from build123d import *

# Parameters (mm, degrees)
SKETCH1_R           = 65
SKETCH1_R_2         = 3.75
SKETCH1_R_3         = 2.25
BOSS_EXTRUDE1_DEPTH = 2.3749


with BuildPart() as part:
    # Sketch1 → Boss-Extrude1 (new, symmetric)
    with BuildSketch(Plane.XY):
        with BuildLine():
            Line((-45.414170693, 71.792048343), (-34.829629131, 111.294095226))
            ThreePointArc((-34.829629131, 111.294095226), (-33.043807145, 113.966766701), (-30, 115))
            Line((-30, 115), (30, 115))
            ThreePointArc((30, 115), (33.043807145, 113.966766701), (34.829629131, 111.294095226))
            Line((34.829629131, 111.294095226), (45.414170693, 71.792048343))
            ThreePointArc((45.414170693, 71.792048343), (46.806677386, 68.753444104), (49.122761322, 66.343476093))
            ThreePointArc((49.122761322, 66.343476093), (82.55, 0), (49.122761322, -66.343476093))
            ThreePointArc((49.122761322, -66.343476093), (46.806677386, -68.753444104), (45.414170693, -71.792048343))
            Line((45.414170693, -71.792048343), (34.829629131, -111.294095226))
            ThreePointArc((34.829629131, -111.294095226), (33.043807145, -113.966766701), (30, -115))
            Line((30, -115), (-30, -115))
            ThreePointArc((-30, -115), (-33.043807145, -113.966766701), (-34.829629131, -111.294095226))
            Line((-34.829629131, -111.294095226), (-45.414170693, -71.792048343))
            ThreePointArc((-45.414170693, -71.792048343), (-46.806677386, -68.753444104), (-49.122761322, -66.343476093))
            ThreePointArc((-49.122761322, -66.343476093), (-82.55, 0), (-49.122761322, 66.343476093))
            ThreePointArc((-49.122761322, 66.343476093), (-46.806677386, 68.753444104), (-45.414170693, 71.792048343))
        make_face()
        Circle(SKETCH1_R, mode=Mode.SUBTRACT)
        with Locations((-20, 100)):
            Circle(SKETCH1_R_2, mode=Mode.SUBTRACT)
        with Locations((20, 100)):
            Circle(SKETCH1_R_2, mode=Mode.SUBTRACT)
        with Locations(Location((20, -100, 0), (0, 0, 180))):
            Circle(SKETCH1_R_2, mode=Mode.SUBTRACT)
        with Locations(Location((-20, -100, 0), (0, 0, 180))):
            Circle(SKETCH1_R_2, mode=Mode.SUBTRACT)
        with Locations((0, 78.74)):
            Circle(SKETCH1_R_3, mode=Mode.SUBTRACT)
        with Locations((46.282210766, 63.701998137)):
            Circle(SKETCH1_R_3, mode=Mode.SUBTRACT)
        with Locations((74.886190093, 24.331998137)):
            Circle(SKETCH1_R_3, mode=Mode.SUBTRACT)
        with Locations((74.886190093, -24.331998137)):
            Circle(SKETCH1_R_3, mode=Mode.SUBTRACT)
        with Locations((46.282210766, -63.701998137)):
            Circle(SKETCH1_R_3, mode=Mode.SUBTRACT)
        with Locations((0, -78.74)):
            Circle(SKETCH1_R_3, mode=Mode.SUBTRACT)
        with Locations((-46.282210766, -63.701998137)):
            Circle(SKETCH1_R_3, mode=Mode.SUBTRACT)
        with Locations((-74.886190093, -24.331998137)):
            Circle(SKETCH1_R_3, mode=Mode.SUBTRACT)
        with Locations((-74.886190093, 24.331998137)):
            Circle(SKETCH1_R_3, mode=Mode.SUBTRACT)
        with Locations((-46.282210766, 63.701998137)):
            Circle(SKETCH1_R_3, mode=Mode.SUBTRACT)
    extrude(amount=BOSS_EXTRUDE1_DEPTH, both=True)


solid = part.part
Read the model definition and answer for the solid it produces. Units are mm, in the model's axes. Coordinates: 2 decimals unless noted, no trailing zeros. Loops run counter-clockwise (first coordinate to the right, second up) from the corner with the lowest first, then second, coordinate; pieces in that order, holes last. Notation, with made-up numbers: (11.5, -28) - (58.5, -28) arc R29 ccw to (58.5, -3) - close; hole circle Ø3 at (16.5, 34). An arc over 180 degrees is marked (long way). Answer in a Markdown table with one row per item.
Q1. Find section B-B on x = 20. Write down the section's boundary in (y, z), plus the area to 3 significant figures.
Here are the results:
| item | result |
|---|---|
| outline | (-115, -2.37) - (-103.75, -2.37) - (-103.75, 2.37) - (-115, 2.37) - close; (-96.25, -2.37) - (-61.85, -2.37) - (-61.85, 2.37) - (-96.25, 2.37) - close; (61.85, -2.37) - (96.25, -2.37) - (96.25, 2.37) - (61.85, 2.37) - close; (103.75, -2.37) - (115, -2.37) - (115, 2.37) - (103.75, 2.37) - close |
| area | 434 mm^2 |
Q2. Straight lines are drawn through the part: line 1 along Y through (x, z) = (-20, 1.05); line 2 along Y through (x, z) = (0, -0.8); line 3 along Y through (x, z) = (75, -1.6). For each, find the intervals that lie inside material, in ascending order. Write a range as [from, to].
Here are the results:
| item | result |
|---|---|
| line 1 | y = [-115, -103.75], [-96.25, -61.85], [61.85, 96.25], [103.75, 115] |
| line 2 | y = [-115, -80.99], [-76.49, -65], [65, 76.49], [80.99, 115] |
| line 3 | y = [-34.49, -26.58], [-22.08, 22.08], [26.58, 34.49] |
Q3. Find section A-A on y = 0. Write down the section's boundary in (x, z).
Here are the results:
| item | result |
|---|---|
| outline | (-82.55, -2.37) - (-65, -2.37) - (-65, 2.37) - (-82.55, 2.37) - close; (65, -2.37) - (82.55, -2.37) - (82.55, 2.37) - (65, 2.37) - close |
Q4. Find section C-C on y = -100. Write down the section's boundary in (x, z), plus the area to 3 significant figures.
Here are the results:
| item | result |
|---|---|
| outline | (-37.86, -2.37) - (-23.75, -2.37) - (-23.75, 2.37) - (-37.86, 2.37) - close; (-16.25, -2.37) - (16.25, -2.37) - (16.25, 2.37) - (-16.25, 2.37) - close; (23.75, -2.37) - (37.86, -2.37) - (37.86, 2.37) - (23.75, 2.37) - close |
| area | 288 mm^2 |
Q5. Find section D-D on z = -0.2. Count the separate pieces of the cut face and the enclosed holes in it, plus the area to 3 significant figures.
Here are the results:
| item | result |
|---|---|
| separate pieces | 1 |
| enclosed holes | 15 |
| area | 13,500 mm^2 |
Q6. The mould has two halves that part along Y. Classify faces 1 (the cylindrical face through (19.512, 103.718, -0.033)), 2 (the cylindrical face through (-46.575, 65.933, -0.033)), 3 (the cylindrical face through (-46.78, -68.79, 0.03)), 4 (the cylindrical face through (-82.543, -1.079, 0.033)): pulls with the +Y half, pulls with the -Y half, needs draft (parallel to the pull), parting line crosses it, or undercut.
Here are the results:
| item | result |
|---|---|
| face 1 | undercut |
| face 2 | undercut |
| face 3 | pulls with the -Y half |
| face 4 | parting line crosses it |
Q7. Given P1, Ø4, axis at x = 0, y = 78.74, coming from the +Z side; P2, Ø2, axis at y = -66.5, z = 0, coming from the +X side, each flat-ended and moving along its own axis, determine where each tip first touches the part or whether it passes through.
Here are the results:
| item | result |
|---|---|
| P1 | passes through |
| P2 | stops at x = 50.24 |
